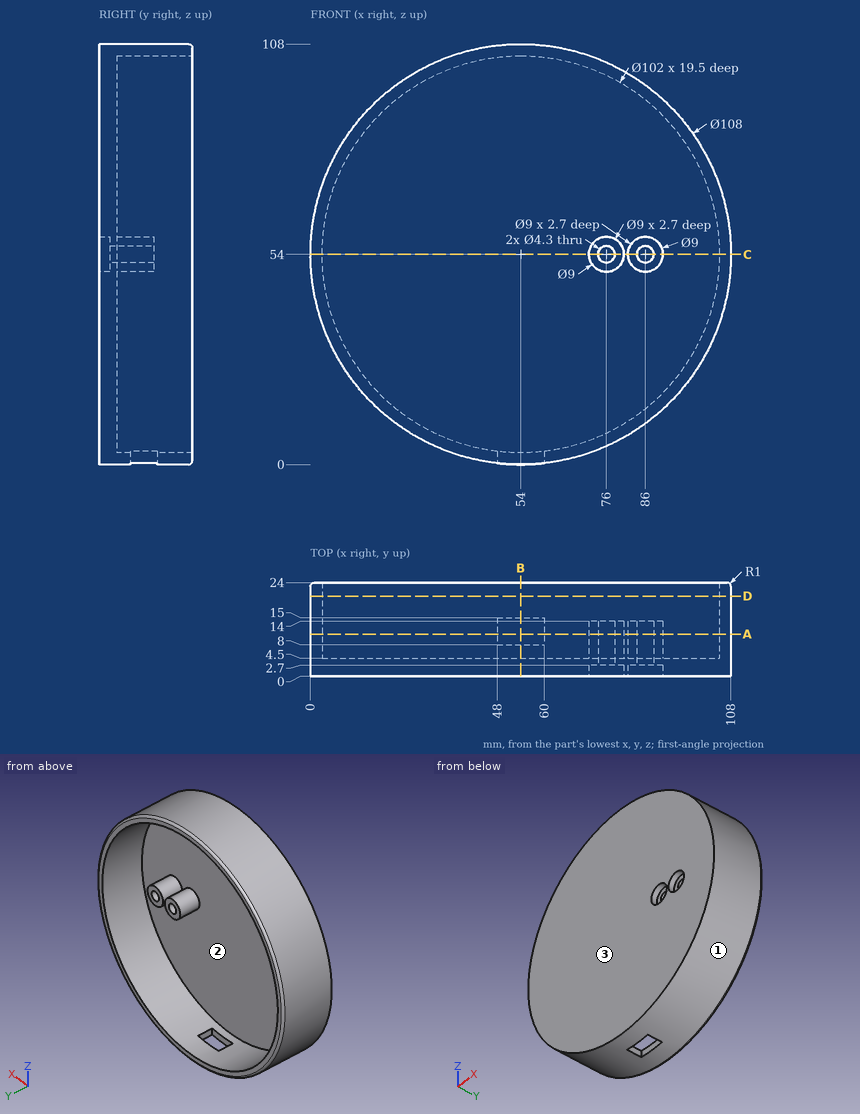
Verification items for this drawing (mm, ordinates from the low corner). Give positions to 0.01 mm unless a question says otherwise; leave off trailing zeros. Loops run counter-clockwise (first coordinate to the right, second up) from the corner with the lowest first, then second, coordinate; pieces in that order, holes last. Notation, with made-up numbers: M 76,15.25 L 82,15.25 A13 ccw 82,30.25 Z; hole C 74,88 d4. An arc over 180 degrees is marked long. Answer as a JSON object with one key per item and string values. Group by question number.
Q1. Cross-section at D-D on y = 20.5. Record the cut outline in (x, z).
Q2. Cross-section at A-A on y = 10.75. Record the cut outline in (x, z).
Q3. Release check for a two-part mould opening along X. For the marked faces 1, 2 and 3 record: released by +X, released by -X, zero draft, split by the parting line, or undercut.
Q4. Cross-section at C-C on z = 54. Give the number of separate pieces and of enclosed holes in the cut face, then the cut area to 3 significant figures.
Q5. Go/stop test with flat-tipped pins: P1, Ø8, axis at x = 86, z = 54, coming from the -Y side; P2, Ø4, axis at y = 11.5, z = 27, coming from the -X side; P3, Ø2, axis at y = 12.5, z = 82.5, coming from the -X side. Record where each tip stops, or that it passes through.
Q6. Cross-section at B-B on x = 54. Record the cut outline in (y, z).
Q7. Material ranges on line 1 along X through (y, z) = (1, 54); line 2 along X through (y, z) = (6.25, 54); line 3 along Y through (x, z) = (74, 64.5), recorded low to high. Write a range as [from, to].
Evaluation:
{
 "1": {"outline": "C 54,54 d108; hole C 54,54 d102"},
 "2": {"outline": "M 48,0.33 L 48,3.35 A51 cw long 60,3.35 L 60,0.33 A54 ccw long Z; C 76,54 d9; C 86,54 d9; hole C 76,54 d4.3; hole C 86,54 d4.3"},
 "3": {"face 1": "split by the parting line", "face 2": "undercut", "face 3": "zero draft"},
 "4": {"separate pieces": "3", "enclosed holes": "0", "area": "628 mm2"},
 "5": {"P1": "stops at y = 2.7", "P2": "stops at x = 6.14", "P3": "stops at x = 7.53"},
 "6": {"outline": "M 0,0 L 8,0 L 8,3 L 4.5,3 L 4.5,105 L 24,105 L 24,107 A1 ccw 23,108 L 0,108 Z; M 15,0 L 23,0 A1 ccw 24,1 L 24,3 L 15,3 Z"},
 "7": {"line 1": "x = [0, 71.5], [80.5, 81.5], [90.5, 108]", "line 2": "x = [0, 3], [71.5, 73.85], [78.15, 80.5], [81.5, 83.85], [88.15, 90.5], [105, 108]", "line 3": "y = [0, 4.5]"}
}
